Geometry: final body of the model. Coordinates: model frame, mm. A direction names the side the tool comes from. Give positions to 0.01 mm unless a question says otherwise; leave off trailing zeros. Write each loop counter-clockwise with the first axis right and the second up, starting at its lowest first coordinate (ties: lowest second). Pieces come first, ordered by that corner, then holes.
Q1. Mould query, pull axis Z, two halves, no side actions, for faces 4 (the cylindrical face through (-30.29, 49.18, -1.76)), 5 (the flat face through (11.837, -12, 12)), 6 (the flat face through (18.985, 11, -4)). Classes: +Z half, -Z half, draft (parallel to the pull), parting line (faces both ways), or undercut.
Q2. Section B-B (y = -24.5). Return the cut outline in (x, z).
Q3. Reachability of faces 1 (the flat face through (-74.163, 28, 8)), 2 (the flat face through (-84.663, 9, 0)), 3 (the cylindrical face through (13.44, 45.47, 0.68)) from +Z, -Z, +X, -X, +Y, -Y: full face, straight path, thin tool, end or side. Return the list, or none.
Q4. Section C-C (x = 30.5). Return the cut outline in (y, z), plus the area to 3 significant figures.
Q5. Section A-A (z = 0). Return the cut outline in (x, y), plus the area to 3 significant figures.
Q6. Line query: line 1 (X direction, y = -27, z = 11); line 2 (X direction, y = 31, z = 9.5); line 3 (Z direction, x = -63, y = 1). Output: solid intervals per line, ascending.
Q7. Section D-D (z = -24). Return the cut outline in (x, y), plus the area to 3 significant figures.
Q8. Pin query (flat end, axial travel): pin 1 Ø12 at (x, y) = (-16, 19) entering from +Z; pin 2 Ø11.5 at (y, z) = (-23.5, -2.5) entering from +X; pin 3 Ø1 at (x, y) = (-10, 7) entering from +Z. Return the tip coordinate at first contact, or that it passes through.
from build123d import *

# Parameters (mm, degrees)
SKETCH1_W          = 10.5
SKETCH1_H          = 20
SKETCH1_W_2        = 73.726566952
SKETCH1_H_2        = 40
SKETCH1_W_3        = 20
SKETCH1_H_3        = 4
SKETCH4_R          = 5.236569571
CUT_EXTRUDE3_DEPTH = 3
SKETCH7_R          = 4
CUT_EXTRUDE4_DEPTH = 3


with BuildPart() as part:
    # Sketch1 → Revolve2 (revolve)
    with BuildSketch(Plane.XY, mode=Mode.PRIVATE) as revolve2_sk:
        with Locations((-79.413135593, 19.219422603)):
            Rectangle(SKETCH1_W, SKETCH1_H)
        Polygon((-66.795719354, 49.219422603), (-74.163135593, 49.219422603), (-74.163135593, 29.219422603), (-74.163135593, 9.219422603), (-66.795719354, 9.219422603), align=None)
        with Locations((-29.932435878, 29.219422603)):
            Rectangle(SKETCH1_W_2, SKETCH1_H_2)
        Polygon((14.836864407, 49.219422603), (6.930847598, 49.219422603), (6.930847598, 9.219422603), (14.836864407, 9.219422603), (14.836864407, 17.219422603), align=None)
        Polygon((18.985169492, 17.219422603), (14.836864407, 17.219422603), (14.836864407, 9.219422603), (18.985169492, 9.219422603), (18.985169492, 13.219422603), align=None)
        with Locations((28.985169492, 11.219422603)):
            Rectangle(SKETCH1_W_3, SKETCH1_H_3)
    revolve(revolve2_sk.sketch.rotate(Axis((-107.444319021, 9.219422603, 0), (1, 0, 0)), 180), axis=Axis((-107.444319021, 9.219422603, 0), (1, 0, 0)))

    # Sketch4 → Cut-Extrude3 (cut)
    with BuildSketch(Plane(origin=(15, 0, 0), x_dir=(0, 0, -1), z_dir=(1, 0, 0))):
        with Locations((0, 40.278768816)):
            Circle(SKETCH4_R)
        with Locations(Location((0, -21.839923611, 0), (0, 0, 90))):
            Circle(SKETCH4_R)
    extrude(amount=-CUT_EXTRUDE3_DEPTH, mode=Mode.SUBTRACT)

    # Sketch7 → Cut-Extrude4 (cut)
    with BuildSketch(Plane(origin=(14.836864407, 0, 0), x_dir=(0, 0, -1), z_dir=(1, 0, 0))):
        with Locations(Location((-11.762505522, -11.700507222, 0), (0, 0, 90))):
            Circle(SKETCH7_R)
        with Locations(Location((-12, 30.004032293, 0), (0, 0, 90))):
            Circle(SKETCH7_R)
        with Locations(Location((24, 9.219422603, 0), (0, 0, 90))):
            Circle(SKETCH7_R)
    extrude(amount=-CUT_EXTRUDE4_DEPTH, mode=Mode.SUBTRACT)


solid = part.part
Computed:
1. face 4: parting line
1. face 5: undercut
1. face 6: draft
2. outline: (-74.16, -21.52) - (14.84, -21.52) - (14.84, -4.51) - (12, -4.51) - (12, 4.51) - (14.84, 4.51) - (14.84, 21.52) - (-74.16, 21.52) - close
3. face 1: -X
3. face 2: +Z, -Z, -X, +Y, -Y
3. face 3: +X
4. outline: circle Ø8 at (9.22, 0)
4. area: 50.3 mm2
5. outline: (-84.66, -10.78) - (-74.16, -10.78) - (-74.16, -30.78) - (14.84, -30.78) - (14.84, -27.08) - (12, -27.08) - (12, -16.6) - (14.84, -16.6) - (14.84, 1.22) - (18.99, 1.22) - (18.99, 5.22) - (38.99, 5.22) - (38.99, 13.22) - (18.99, 13.22) - (18.99, 17.22) - (14.84, 17.22) - (14.84, 35.04) - (12, 35.04) - (12, 45.52) - (14.84, 45.52) - (14.84, 49.22) - (-74.16, 49.22) - (-74.16, 29.22) - (-84.66, 29.22) - close
5. area: 7,710 mm2
6. line 1: x = -74.16 to 14.84
6. line 2: x = -74.16 to 11.84
6. line 3: z = -39.15 to 39.15
7. outline: (-74.16, -22.78) - (14.84, -22.78) - (14.84, 5.22) - (11.84, 5.22) - (11.84, 13.22) - (14.84, 13.22) - (14.84, 41.22) - (-74.16, 41.22) - close
7. area: 5,670 mm2
8. pin 1: stops at z = 39.82
8. pin 2: stops at x = 14.84
8. pin 3: stops at z = 39.96
